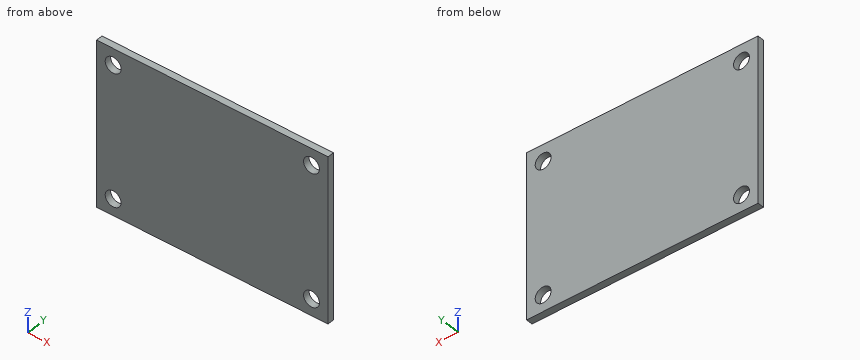
from build123d import *

# Parameters (mm, degrees)
SKICA2_W                 = 35
SKICA2_H                 = 25
P_IDAT_VYSUNUT_M1_DEPTH  = 1
SKICA3_R                 = 1.2
ODEBRAT_VYSUNUT_M1_DEPTH = 1
LINPOLE1_COUNT           = 2
LINPOLE1_PITCH           = 30
LINPOLE1_COUNT_DIR2      = 2
LINPOLE1_PITCH_DIR2      = 20


with BuildPart() as part:
    # Skica2 → Přidat vysunutím1 (new body)
    with BuildSketch(Plane(origin=(0, 0, 0), x_dir=(1, 0, 0), z_dir=(0, 1, 0))):
        Rectangle(SKICA2_W, SKICA2_H)
    extrude(amount=P_IDAT_VYSUNUT_M1_DEPTH)

    # Skica3 → Odebrat vysunutím1 (cut)
    with BuildSketch(Plane(origin=(0, 1, 0), x_dir=(1, 0, 0), z_dir=(0, 1, 0))):
        with Locations((-15, 10)):
            Circle(SKICA3_R)
    odebrat_vysunut_m1 = extrude(amount=-ODEBRAT_VYSUNUT_M1_DEPTH, mode=Mode.SUBTRACT)

    # LinPole1: Odebrat vysunut_m1 2 × 2
    with Locations(*[(i * LINPOLE1_PITCH, 0, j * LINPOLE1_PITCH_DIR2) for i in range(LINPOLE1_COUNT) for j in range(LINPOLE1_COUNT_DIR2) if (i, j) != (0, 0)]):
        add(odebrat_vysunut_m1, mode=Mode.SUBTRACT)


solid = part.part
CAD build for the part. Positions are in the model's coordinates, mm. Coordinates: 2 decimals unless noted, no trailing zeros. Write each loop counter-clockwise with the first axis right and the second up, starting at its lowest first coordinate (ties: lowest second). Pieces come first, ordered by that corner, then holes. Notation, with made-up numbers: (72.25, 10.25) - (119.25, 10.25) arc R13 ccw to (119.25, 32.25) - close; hole circle Ø9 at (-28, 68). An arc over 180 degrees is marked (long way). Use a Markdown table: item, result. Add a question column.
Item 1: Flat gauge pin, fed straight in: pin 1 (4 mm diameter, centred on x = -15, z = -10, fed in from +Y). Where does the tip first touch, or does it go through?
Item 2: Band-saw the part on C-C, the plane y = 0.45. Give the cut face in (x, z), and give its area (3 significant figures).
Item 3: Band-saw the part on B-B, the plane x = 15. Give the cut face in (y, z).
Item 4: Drill centre lines: L1, parallel to Z at x = -15, y = 0.8; L2, parallel to X at y = 0.4, z = 10; L3, parallel to Z at x = -14.5, y = 0.6. Where is each one in solid material? Low to high. Write a range as from..to.
Item 5: Band-saw the part on A-A, the plane z = -10. Give the cut face in (x, y), and give its area (3 significant figures).
Numbers:
| question | item | result |
|---|---|---|
| 1 | pin 1 | y = 1 |
| 2 | outline | (-17.5, -12.5) - (17.5, -12.5) - (17.5, 12.5) - (-17.5, 12.5) - close; hole circle Ø2.4 at (-15, -10); hole circle Ø2.4 at (-15, 10); hole circle Ø2.4 at (15, -10); hole circle Ø2.4 at (15, 10) |
| 2 | area | 857 mm2 |
| 3 | outline | (0, -12.5) - (1, -12.5) - (1, -11.2) - (0, -11.2) - close; (0, -8.8) - (1, -8.8) - (1, 8.8) - (0, 8.8) - close; (0, 11.2) - (1, 11.2) - (1, 12.5) - (0, 12.5) - close |
| 4 | L1 | -12.5..-11.2, -8.8..8.8, 11.2..12.5 |
| 4 | L2 | -17.5..-16.2, -13.8..13.8, 16.2..17.5 |
| 4 | L3 | -12.5..-11.09, -8.91..8.91, 11.09..12.5 |
| 5 | outline | (-17.5, 0) - (-16.2, 0) - (-16.2, 1) - (-17.5, 1) - close; (-13.8, 0) - (13.8, 0) - (13.8, 1) - (-13.8, 1) - close; (16.2, 0) - (17.5, 0) - (17.5, 1) - (16.2, 1) - close |
| 5 | area | 30.2 mm2 |
